```python
from build123d import *

# Parameters (mm, degrees)
MAINBLOCK_R                     = 2
MAINBLOCKBOSS_EXTRUDE1_DEPTH    = 23.4
TOPHOLECUT_SKETCH2_R            = 2.5
TOPHOLECUT_EXTRUDE1_DEPTH       = 45
TOPSPACERSKETCH4_R              = 3.5
TOPSPACERSKETCH4_R_2            = 2.5
TOPSPACERBOSS_EXTRUDE2_DEPTH    = 1
LOWERSPACERBOSS_EXTRUDE3_START  = 1
LOWERSPACERSKETCH5_R            = 3.5
LOWERSPACERSKETCH5_R_2          = 2.5
LOWERSPACERBOSS_EXTRUDE3_DEPTH  = 1
MOUNTHOLEBORECUT_EXTRUDE1_DEPTH = 2
PUSHPINHOLESKETCH1_R            = 1
PUSHPINHOLECUT_EXTRUDE1_DEPTH   = 76.354665582
SCREWCOLLISIONSKETCH1_W         = 18.72
SCREWCOLLISIONSKETCH1_H         = 60
CUT_EXTRUDE1_DEPTH              = 5
FILLET1_R                       = 10
FILLET2_R                       = 10
MIDRAILINSETSKETCH1_W           = 3.18
MIDRAILINSETSKETCH1_H           = 40.4
MIDRAILINSETCUT_EXTRUDE2_DEPTH  = 76.354665582


with BuildPart() as part:
    # MainBlock → MainBlockBoss-Extrude1 (new body)
    with BuildSketch(Plane.XY):
        Polygon((0, 0), (39.125, 0), (39.125, 19.8), (19.725, 19.8), (19.725, 40.2), (39.125, 40.2), (39.125, 60), (0, 60), align=None)
        with Locations((11.1125, 50.1)):
            Circle(MAINBLOCK_R, mode=Mode.SUBTRACT)
        with Locations((11.1125, 9.9)):
            Circle(MAINBLOCK_R, mode=Mode.SUBTRACT)
    extrude(amount=MAINBLOCKBOSS_EXTRUDE1_DEPTH)

    # TopHoleCut-Sketch2 → TopHoleCut-Extrude1 (cut)
    with BuildSketch(Plane(origin=(0, 60, 0), x_dir=(1, 0, 0), z_dir=(0, 1, 0))):
        with Locations(Location((29.425, -11.7, 0), (0, 0, 270))):
            Circle(TOPHOLECUT_SKETCH2_R)
    extrude(amount=-TOPHOLECUT_EXTRUDE1_DEPTH, mode=Mode.SUBTRACT)

    # TopSpacerSketch4 → TopSpacerBoss-Extrude2 (add)
    with BuildSketch(Plane.XZ.offset(-40.2)):
        with Locations(Location((29.425, 11.7, 0), (0, 0, 90))):
            Circle(TOPSPACERSKETCH4_R)
        with Locations(Location((29.425, 11.7, 0), (0, 0, 90))):
            Circle(TOPSPACERSKETCH4_R_2, mode=Mode.SUBTRACT)
    extrude(amount=TOPSPACERBOSS_EXTRUDE2_DEPTH)

    # LowerSpacerSketch5 → LowerSpacerBoss-Extrude3 (add)
    with BuildSketch(Plane(origin=(0, 19.8, 0), x_dir=(1, 0, 0), z_dir=(0, 1, 0)).offset(LOWERSPACERBOSS_EXTRUDE3_START)):
        with Locations(Location((29.425, -11.7, 0), (0, 0, 270))):
            Circle(LOWERSPACERSKETCH5_R)
        with Locations(Location((29.425, -11.7, 0), (0, 0, 270))):
            Circle(LOWERSPACERSKETCH5_R_2, mode=Mode.SUBTRACT)
    extrude(amount=-LOWERSPACERBOSS_EXTRUDE3_DEPTH)

    # MountHoleBoreSketch1 → MountHoleBoreCut-Extrude1 (cut)
    with BuildSketch(Plane(origin=(0, 0, 0), x_dir=(-1, 0, 0), z_dir=(0, 0, -1))):
        Polygon((-7.2375, 50.1), (-9.175, 53.45584844), (-13.05, 53.45584844), (-14.9875, 50.1), (-13.05, 46.74415156), (-9.175, 46.74415156), align=None)
        Polygon((-7.2375, 9.9), (-9.175, 13.25584844), (-13.05, 13.25584844), (-14.9875, 9.9), (-13.05, 6.54415156), (-9.175, 6.54415156), align=None)
    extrude(amount=-MOUNTHOLEBORECUT_EXTRUDE1_DEPTH, mode=Mode.SUBTRACT)

    # PushPinHoleSketch1 → PushPinHoleCut-Extrude1 (cut, through all)
    with BuildSketch(Plane.XZ):
        with Locations(Location((29.425, 11.7, 0), (0, 0, 270))):
            Circle(PUSHPINHOLESKETCH1_R)
    extrude(amount=-PUSHPINHOLECUT_EXTRUDE1_DEPTH, mode=Mode.SUBTRACT)

    # ScrewCollisionSketch1 → Cut-Extrude1 (cut)
    with BuildSketch(Plane.ZY):
        with Locations((14.04, 30)):
            Rectangle(SCREWCOLLISIONSKETCH1_W, SCREWCOLLISIONSKETCH1_H)
    extrude(amount=-CUT_EXTRUDE1_DEPTH, mode=Mode.SUBTRACT)

    # Fillet1
    # the kernel refuses this fillet: 10 mm, written as the material it adds along each edge
    with BuildSketch(Plane(origin=(5, 60, 4.68), x_dir=(0, 0, 1), z_dir=(0, -1, 0))) as fillet1_piece_1:
        with BuildLine():
            CenterArc((8.660254038, 10), FILLET1_R, 210, 60)
            Line((0, 5), (-0.173205081, 4.9))
            ThreePointArc((-0.173205081, 4.9), (-0.2, 2.5), (-0.2, 0))
            Line((-0.2, 0), (0, -0.2))
            Line((0, -0.2), (8.660254038, -0.2))
            Line((8.660254038, -0.2), (8.660254038, 0))
        make_face()
    extrude(amount=60)

    # Fillet2
    fillet2_edges = [part.edges().sort_by_distance(p)[0] for p in [
        (0, 30, 4.68),
    ]]
    fillet(fillet2_edges, radius=FILLET2_R)

    # MidRailInsetSketch1 → MidRailInsetCut-Extrude2 (cut, through all)
    with BuildSketch(Plane(origin=(0, 0, 0), x_dir=(-1, 0, 0), z_dir=(0, 0, -1))):
        with Locations((-1.59, 20.2)):
            Rectangle(MIDRAILINSETSKETCH1_W, MIDRAILINSETSKETCH1_H)
    extrude(amount=-MIDRAILINSETCUT_EXTRUDE2_DEPTH, mode=Mode.SUBTRACT)


solid = part.part
```
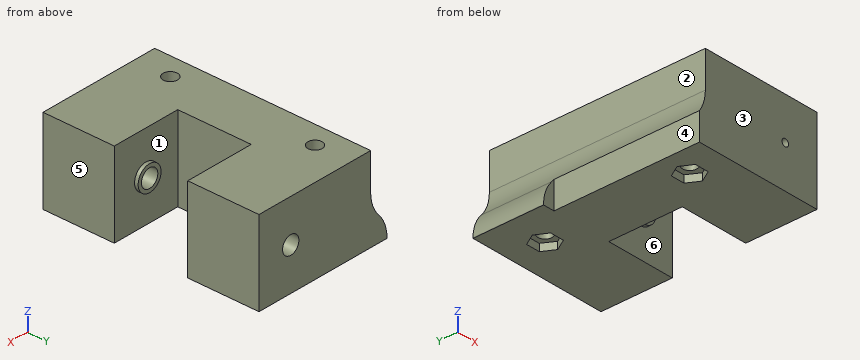
Geometry check sheet. Reference: the model listing, model coordinates, mm. Face numbers are marked on the shaded views. A direction names the side the tool comes from. Round coordinates to 2 decimals unless told otherwise and drop trailing zeros. Order: outer loops, then holes, each group sorted by start corner. A loop starts at its lowest first (then second) coordinate and runs counter-clockwise, first axis right, second up. Notation, with made-up numbers: M 55,56 L 67,56 A22 ccw 67,64 Z; hole C 73,6 d5. An arc over 180 degrees is marked long. Answer as CSV lines item,"result".
1) Mould release check, pull along Y, two halves, no side actions. Record for the marked faces 1, 2 and 3: +Y half, -Y half, draft (parallel to the pull), parting line (faces both ways), or undercut.
Entries:
face 1,"undercut"
face 2,"draft"
face 3,"-Y half"
2) Thickness scan on probe 1 along Y at (x, z) = (21.5, 6); probe 2 along X at (y, z) = (9, 11.7) (3 decimals); probe 3 along Y at (x, z) = (12, 13.25). Record the ranges inside material, lowest first. Write a range as [from, to].
Entries:
probe 1,"[0, 19.8], [40.2, 60]"
probe 2,"[4.865, 9.326], [12.899, 28.425], [30.425, 39.125]"
probe 3,"[0, 8.11], [11.69, 48.31], [51.89, 60]"
3) Tool access check on the marked faces 4, 5 and 6. Record the directions out of +Z, -Z, +X, -X, +Y, -Y that give a thin tool (end or side, any length) a straight path to the whole face; none if there is none.
Entries:
face 4,"+Z, -Z, -X, -Y"
face 5,"+Z, -Z, +X, +Y, -Y"
face 6,"none"
4) Gauge pin test, flat ends, axial feed: pin 1 Ø12 at (y, z) = (31, 9) entering from +X (3 decimals); pin 2 Ø10 at (y, z) = (44.5, 5.5) entering from -X; pin 3 Ø3 at (y, z) = (42.5, 13.5) entering from -X; pin 4 Ø1 at (x, y) = (10.5, 11) entering from +Z. Record the tip position at first contact, or that the pin passes through.
Entries:
pin 1,"x = 19.725"
pin 2,"x = 0.01"
pin 3,"x = 4.91"
pin 4,"through"
5) Sectioned sample at B-B on z = 18.75. Record the cut outline in (x, y) (1 decimal), and give its area (3 significant figures).
Entries:
outline,"M 5,0 L 39.1,0 L 39.1,19.8 L 19.7,19.8 L 19.7,40.2 L 39.1,40.2 L 39.1,60 L 5,60 Z; hole C 11.1,9.9 d4; hole C 11.1,50.1 d4"
area,"1,630 mm2"
6) Sectioned sample at A-A on x = 11.5. Record the cut outline in (y, z), and give its area (3 significant figures).
Entries:
outline,"M 0,0 L 6.54,0 L 6.54,2 L 7.94,2 L 7.94,23.4 L 0,23.4 Z; M 11.86,2 L 13.26,2 L 13.26,0 L 46.74,0 L 46.74,2 L 48.14,2 L 48.14,23.4 L 11.86,23.4 Z; M 52.06,2 L 53.46,2 L 53.46,0 L 60,0 L 60,23.4 L 52.06,23.4 Z"
area,"1,210 mm2"
7) Sectioned sample at C-C on y = 49. Give the number of separate pieces and of enclosed holes in the cut face, and give its area (3 significant figures).
Entries:
separate pieces,"2"
enclosed holes,"1"
area,"728 mm2"
